Design review of the part built by this model. Coordinates are the model's own, in mm. Face numbers are marked on the shaded views. A direction names the side the tool comes from. Coordinates: 2 decimals unless noted, no trailing zeros. Order: outer loops, then holes, each group sorted by start corner. A loop starts at its lowest first (then second) coordinate and runs counter-clockwise, first axis right, second up. Notation, with made-up numbers: M 56.5,21 L 81.5,21 A19 cw 81.5,41 Z; hole C 3.25,71 d2. An arc over 180 degrees is marked long. Answer as a JSON object with one key per item and string values.
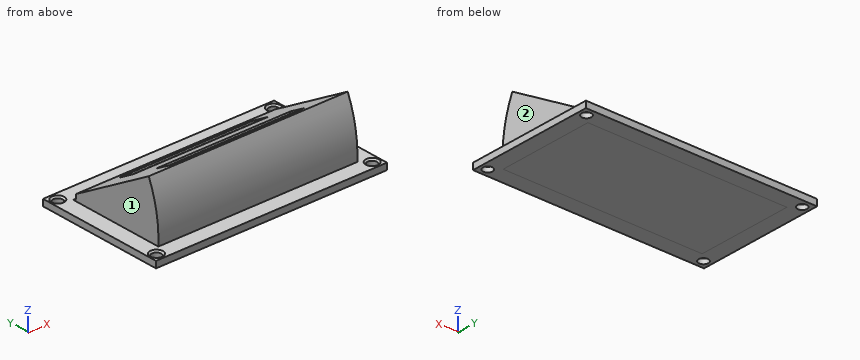
Autodesk Inventor part; units mm, degrees
ref_plane "YZ Plane" through (0, 0, 0) normal (1, 0, 0) x (0, 1, 0)
ref_plane "XZ Plane" through (0, 0, 0) normal (0, 1, 0) x (-1, 0, 0)
ref_plane "XY Plane" through (0, 0, 0) normal (0, 0, 1) x (1, 0, 0)
sketch "Sketch1" plane through (0, 0, 0) normal (0, 0, 1) x (1, 0, 0)
  line L0 (0, 0) -> (62, 0)
  line L1 (62, 0) -> (62, 30)
  line L2 (62, 30) -> (0, 30)
  line L3 (0, 30) -> (0, 0)
  dimension "d0" = 62
  dimension "d1" = 30
sketch "Sketch2" plane through (0, 0, 0) normal (1, 0, 0) x (0, 1, 0)
  line L0 (0, 0) -> (30, 0)
  arc A0 (16.1062, 11.6791) -> (15, 0) centre (36.6604, 3.8403) ccw
sweep "Sweep1" add profiles "Sketch1" path "Sketch2" path curves A0
sketch "Sketch3" plane through (62, 0, 0) normal (0, 0, -1) x (-1, 0, 0)
  line L0 (0, 0) -> (0, 30)
  line L1 (62, 0) -> (0, 0)
  line L2 (62, 30) -> (62, 0)
  line L3 (0, 30) -> (62, 30)
  line L4 (0, 30) -> (62, 0) construction
  line L5 (0, 0) -> (62, 30) construction
  line L6 (67, 35) -> (67, -5)
  line L7 (67, -5) -> (-5, -5)
  line L8 (-5, -5) -> (-5, 35)
  line L9 (-5, 35) -> (67, 35)
  dimension "d4" = 5
extrude "Extrusion1" add sketch "Sketch3" against normal blind 2
sketch "Sketch4" plane through (67, -5, 0) normal (0, 0, -1) x (-1, 0, 0)
  point P0 (67, 5)
sketch "Sketch6" plane through (0, 28.9732, 3.9694) normal (0, 0.514, 0.8578) x (1, 0, 0)
  line L0 (0, 1.893) -> (62, 1.893) construction
  line L1 (62, -30) -> (62, 0) construction
  line L2 (62, -15) -> (0, -15) construction
  line L3 (0, -23.9737) -> (0, -30) construction
  line L4 (31, -15) -> (31, -30) construction
  line L5 (31, -15) -> (31, 0) construction
  line L6 (62, 0) -> (0, 0) construction
  line L7 (62, -22.5) -> (31, -22.5) construction
  line L8 (31, -22.5) -> (0, -22.5) construction
  line L9 (31, -7.5) -> (0, -7.5) construction
  line L10 (0, 0) -> (0, -30) construction
  line L11 (31, -7.5) -> (62, -7.5) construction
  line L12 (51.9742, -19.576) -> (10.0258, -19.576)
  line L13 (10.0258, -19.576) -> (10.0258, -25.424)
  line L14 (10.0258, -25.424) -> (51.9742, -25.424)
  line L15 (51.9742, -25.424) -> (51.9742, -19.576)
  line L16 (51.9742, -19.576) -> (10.0258, -25.424) construction
  line L17 (10.0258, -19.576) -> (51.9742, -25.424) construction
  line L18 (51.9742, -10.424) -> (10.0258, -10.424)
  line L19 (10.0258, -10.424) -> (10.0258, -4.576)
  line L20 (10.0258, -4.576) -> (51.9742, -4.576)
  line L21 (51.9742, -4.576) -> (51.9742, -10.424)
  point P0 (0, -22.8131)
  dimension "d8" = 15
  dimension "d9" = 15
  dimension "d10" = 82.064
  dimension "d11" = 41.9483
extrude "Extrusion2" cut sketch "Sketch6" against normal blind 0.5
sketch "Sketch7" plane through (67, -5, 0) normal (0, 0, -1) x (-1, 0, 0)
  circle A0 centre (2.3883, 37.4725) radius 1.5
  line L0 (72, 40) -> (0, 40) construction
  line L1 (36, 40) -> (36, 0) construction
  line L2 (72, 0) -> (0, 0) construction
  line L3 (0, 40) -> (0, 0) construction
  line L4 (0, 20) -> (72, 20) construction
  line L5 (72, 40) -> (72, 0) construction
  circle A1 centre (2.3883, 2.5275) radius 1.5
  circle A2 centre (69.6117, 37.4725) radius 1.5
  circle A3 centre (69.6117, 2.5275) radius 1.5
  point P0 (67, 5)
  dimension "d14" = 3
extrude "Extrusion3" cut sketch "Sketch7" against normal blind 25.4
chamfer "Chamfer1" distance 0.5 angle 45 4 edges at (-1.1117, -2.4725, 2) (66.1117, -2.4725, 2) (66.1117, 32.4725, 2) (-1.1117, 32.4725, 2)
properties part number "DsholdtilterV1"
1) To check wall thickness, follow L1, parallel to Z at x = 8.5, y = -1.5; L2, parallel to X at y = 1, z = 2.75; L3, parallel to Y at x = 34.5, z = 1.75. State the ranges of each line that lie inside material, in increasing order.
Taken from the geometry:
{"L1": "z = 0 to 2", "L2": "x = 0 to 62", "L3": "y = -5 to 29.26, 30 to 35"}
2) Tool access review of the marked faces 1 and 2: name each direction out of +Z, -Z, +X, -X, +Y, -Y from which nothing blocks a thin tool from reaching the whole face with its end or side.
Taken from the geometry:
{"face 1": "+Z, -X, +Y, -Y", "face 2": "+Z, +X, +Y, -Y"}
3) Add section B-B (y = 17.5). State the section outline as (x, z) points, and give its area (3 significant figures).
Taken from the geometry:
{"outline": "M -5,0 L 67,0 L 67,2 L 62,2 L 62,10.84 L 0,10.84 L 0,2 L -5,2 Z", "area": "692 mm2"}
4) Insertion check: pin 1 Ø1.5 at (y, z) = (19, 9) entering from -X; pin 2 Ø5 at (x, z) = (39, 15.5) entering from -Y; pin 3 Ø8 at (y, z) = (19.5, 16) entering from -X; pin 4 Ø1.7 at (y, z) = (22, 7) entering from +X. Each pin has a flat end and moves straight along its axis. Give the tip position at first contact, or say it passes through.
Taken from the geometry:
{"pin 1": "stops at x = 0", "pin 2": "stops at y = 0.96", "pin 3": "passes through", "pin 4": "stops at x = 62"}
5) Add section C-C (z = 7.25). State the section outline as (x, y) points, and give its area (3 significant figures).
Taken from the geometry:
{"outline": "M 0,-0.04 L 62,-0.04 L 62,23.5 L 51.97,23.5 L 51.97,22.52 L 10.03,22.52 L 10.03,23.5 L 0,23.5 Z", "area": "1,420 mm2"}
